Here's how the part is built. I have some questions about the finished solid (model axes, mm). Face numbers are marked on the shaded views. A direction names the side the tool comes from. Round coordinates to 2 decimals unless told otherwise and drop trailing zeros. Order: outer loops, then holes, each group sorted by start corner. A loop starts at its lowest first (then second) coordinate and runs counter-clockwise, first axis right, second up. Notation, with made-up numbers: (-25.75, 12) -> (17.25, 12) arc R23 cw to (17.25, 24) -> close; hole circle Ø4 at (35.5, 86). An arc over 180 degrees is marked (long way). Use a Markdown table: item, result. Add a question column.
(1) I want a section at A-A, the plane x = -29. Please give me the cut outline in (y, z).
(2) Thinking about a two-plate mould opening in Z: for the marked faces 1, 2 and 3, which applies, pulls with the +Z half, pulls with the -Z half, needs draft (parallel to the pull), parting line crosses it, or undercut?
(3) On a 3-axis mill with a long thin cutter (end or side, diameter ignored), from which of +Z, -Z, +X, -X, +Y, -Y can I reach the whole of each face in a straight line? I mean the marked faces 4 and 5. Say none if no direction works.
(4) I want a section at D-D, the plane x = -35. Please give me the cut outline in (y, z), then the cut area to 3 significant figures.
(5) If I drill on probe 1 along X at (y, z) = (0.25, -15.25); probe 2 along X at (y, z) = (1.15, -14); probe 3 along Z at (x, y) = (-39.25, 0.7), over which ranges is the centre line in solid material (lowest first)?
(6) I want a section at B-B, the plane z = -17.25. Please give me the cut outline in (x, y).
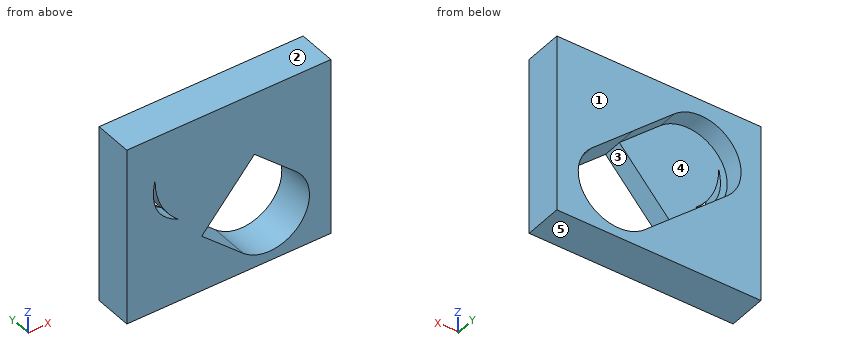
from build123d import *

# Parameters (mm, degrees)
SKETCH1_W           = 16
SKETCH1_H           = 14
BOSS_EXTRUDE1_DEPTH = 3
CUT_EXTRUDE2_DEPTH  = 3
CUT_EXTRUDE3_DEPTH  = 1.5


with BuildPart() as part:
    # Sketch1 → Boss-Extrude1 (new body)
    with BuildSketch(Plane(origin=(0, 0, 0), x_dir=(1, 0, 0), z_dir=(0, 1, 0))):
        with Locations((-34.802547771, 15.318471338)):
            Rectangle(SKETCH1_W, SKETCH1_H)
    extrude(amount=BOSS_EXTRUDE1_DEPTH)

    # Sketch2 → Cut-Extrude2 (cut)
    with BuildSketch(Plane(origin=(0, 3, 0), x_dir=(1, 0, 0), z_dir=(0, 1, 0))):
        with BuildLine():
            Line((-33.679958269, 20.786982613), (-36.931417033, 17.926726524))
            Line((-36.931417033, 17.926726524), (-32.794432226, 13.223918421))
            Line((-32.794432226, 13.223918421), (-29.542973461, 16.08417451))
            ThreePointArc((-29.542973461, 16.08417451), (-29.260061814, 20.504070965), (-33.679958269, 20.786982613))
        make_face()
        with BuildLine():
            add(Edge.make_bspline(
                [(-40.589081196, 11.760287037), (-40.601113462, 14.156732858), (-38.765129592, 15.72931278)],
                knots=[0, 0, 0, 1, 1, 1], degree=2))
            add(Edge.make_bspline(
                [(-38.765129592, 15.72931278), (-40.696042452, 14.851396093), (-40.927669041, 13.342903488), (-40.589081196, 11.760287037)],
                knots=[0, 0, 0, 0, 1, 1, 1, 1], degree=3))
        make_face()
    extrude(amount=-CUT_EXTRUDE2_DEPTH, mode=Mode.SUBTRACT)

    # Sketch3 → Cut-Extrude3 (cut)
    with BuildSketch(Plane(origin=(0, 3, 0), x_dir=(1, 0, 0), z_dir=(0, 1, 0))):
        with BuildLine():
            Line((-32.790440937, 13.219381237), (-36.041899701, 10.359125148))
            ThreePointArc((-36.041899701, 10.359125148), (-40.470324629, 10.642582691), (-40.186867086, 15.071007619))
            Line((-40.186867086, 15.071007619), (-36.935408322, 17.931263708))
            Line((-36.935408322, 17.931263708), (-32.790440937, 13.219381237))
        make_face()
    extrude(amount=-CUT_EXTRUDE3_DEPTH, mode=Mode.SUBTRACT)


solid = part.part
Taken from the geometry:
| question | item | result |
|---|---|---|
| 1 | outline | (0, -22.32) -> (3, -22.32) -> (3, -20.16) -> (0, -20.16) -> close; (0, -16.71) -> (3, -16.71) -> (3, -8.32) -> (0, -8.32) -> close |
| 2 | face 1 | needs draft |
| 2 | face 2 | pulls with the +Z half |
| 2 | face 3 | undercut |
| 3 | face 4 | +Y |
| 3 | face 5 | -Z, +X, -X, +Y, -Y |
| 4 | outline | (0, -22.32) -> (3, -22.32) -> (3, -19.63) -> (0, -19.63) -> close; (0, -15.73) -> (1.5, -15.73) -> (1.5, -11.28) -> (3, -11.28) -> (3, -8.32) -> (0, -8.32) -> close |
| 4 | area | 23.6 mm2 |
| 5 | probe 1 | x = -42.8 to -39.58, -39.26 to -34.58, -30.49 to -26.8 |
| 5 | probe 2 | x = -42.8 to -40.53, -40.12 to -33.48, -31.91 to -26.8 |
| 5 | probe 3 | z = -22.32 to -15.47, -15.27 to -8.32 |
| 6 | outline | (-42.8, 0) -> (-36.34, 0) -> (-36.34, 1.5) -> (-37.71, 1.5) -> (-37.71, 3) -> (-42.8, 3) -> close; (-28.71, 0) -> (-26.8, 0) -> (-26.8, 3) -> (-28.71, 3) -> close |
